Verification items for the finished model (mm, model axes). A direction names the side the tool comes from. Coordinates: 2 decimals unless noted, no trailing zeros. Order: outer loops, then holes, each group sorted by start corner. A loop starts at its lowest first (then second) coordinate and runs counter-clockwise, first axis right, second up. Notation, with made-up numbers: M 57.25,54.5 L 94.25,54.5 A35 cw 94.25,89.5 Z; hole C -3.75,25.5 d7. An arc over 180 degrees is marked long. Answer as a JSON object with one key per item and string values. Group by question number.
(1) Cross-section at A-A (y = 0). Enter the section's corners in (x, z), plus the area to 4 significant figures.
(2) Access from +Z, -Z, +X, -X, +Y, -Y to the whole of each face (thin tool, end or side, straight path). Record for faces 4 (the face through (-6.35, 0, -2)), 5 (the face through (0, -5, 2)), 6 (the face through (2, -6, 0)).
(3) Mould release check, pull along Z, two halves, no side actions. Record for faces 1 (the face through (0, -2, 13)), 2 (the face through (-2, 0, -5)), 3 (the face through (-0.54, -2.44, 8.44)): released by +Z, released by -Z, zero draft, split by the parting line, or undercut.
(4) Gauge pin test, flat ends, axial feed: pin 1 Ø4.5 at (x, y) = (0, 3) entering from +Z; pin 2 Ø8 at (x, z) = (-2, 8) entering from -Y; pin 3 Ø6 at (y, z) = (-3.5, 9) entering from -X; pin 4 Ø1.5 at (y, z) = (1, 6) entering from +X. Record the tip position at first contact, or that the pin passes through.
(5) Cross-section at B-B (x = 0). Enter the section's corners in (y, z), plus the area to 3 significant figures.
(6) Material ranges on line 1 (Y direction, x = 0, z = 11.1); line 2 (Z direction, x = -0.5, y = 4.75); line 3 (Z direction, x = 1.75, y = 6.25), recorded low to high.
(7) Cross-section at C-C (z = 0.75). Enter the section's corners in (x, y), plus the area to 3 significant figures.
from build123d import *

# Parameters (mm, degrees)
EXTRUDE_1_DEPTH     = 5
SKETCH_2_R          = 7.1
EXTRUDE_2_DEPTH     = 2
SKETCH_3_R          = 2.5
EXTRUDE_3_DEPTH     = 7
CHAMFER_1_SIZE      = 2
SKETCH_4_R          = 1.6
CUT_EXTRUDE_1_DEPTH = 30
CHAMFER_2_SIZE      = 1
MOVE_FACE_1_BY      = 4


with BuildPart() as part:
    # ｽｹｯﾁ1 → ﾎﾞｽ - 押し出し1 (new body)
    with BuildSketch(Plane.XY):
        with BuildLine():
            Line((-6.35, -0.875), (-6.036917674, -0.875))
            ThreePointArc((-6.036917674, -0.875), (6.1, 0), (-6.036917674, 0.875))
            Line((-6.036917674, 0.875), (-6.35, 0.875))
            Line((-6.35, 0.875), (-6.35, -0.875))
        make_face()
    extrude(amount=-EXTRUDE_1_DEPTH)

    # ｽｹｯﾁ2 → ﾎﾞｽ - 押し出し2 (add)
    with BuildSketch(Plane.XY):
        Circle(SKETCH_2_R)
    extrude(amount=EXTRUDE_2_DEPTH)

    # ｽｹｯﾁ3 → ﾎﾞｽ - 押し出し3 (add)
    with BuildSketch(Plane.XY.offset(2)):
        Circle(SKETCH_3_R)
    extrude(amount=EXTRUDE_3_DEPTH)

    # 面取り1
    chamfer_1_edges = [part.edges().sort_by_distance(p)[0] for p in [
        (-2.5, 0, 2),
    ]]
    chamfer(chamfer_1_edges, length=CHAMFER_1_SIZE)

    # ｽｹｯﾁ4 → ｶｯﾄ - 押し出し1 (cut)
    with BuildSketch(Plane.XY.offset(9)):
        Circle(SKETCH_4_R)
    extrude(amount=-CUT_EXTRUDE_1_DEPTH, mode=Mode.SUBTRACT)

    # 面取り2
    chamfer_2_edges = [part.edges().sort_by_distance(p)[0] for p in [
        (6.1, 0, -5),
    ]]
    chamfer(chamfer_2_edges, length=CHAMFER_2_SIZE)

    # Move Face 1: a face moved outward by 4.0
    extrude(part.faces().sort_by_distance((0, -2, 9))[0], amount=MOVE_FACE_1_BY, dir=(0, 0, 1))


solid = part.part
Taken from the geometry:
{
 "1": {"outline": "M -7.1,0 L -6.35,0 L -6.35,-5 L -1.6,-5 L -1.6,13 L -2.5,13 L -2.5,4 L -4.5,2 L -7.1,2 Z; M 1.6,-5 L 5.1,-5 L 6.1,-4 L 6.1,0 L 7.1,0 L 7.1,2 L 4.5,2 L 2.5,4 L 2.5,13 L 1.6,13 Z", "area": "91.55 mm²"},
 "2": {"face 4": "-Z, -X, +Y, -Y", "face 5": "+Z", "face 6": "-Z"},
 "3": {"face 1": "released by +Z", "face 2": "released by -Z", "face 3": "zero draft"},
 "4": {"pin 1": "stops at z = 13", "pin 2": "stops at y = -2.5", "pin 3": "stops at x = -2.45", "pin 4": "stops at x = 2.49"},
 "5": {"outline": "M -7.1,0 L -6.1,0 L -6.1,-4 L -5.1,-5 L -1.6,-5 L -1.6,13 L -2.5,13 L -2.5,4 L -4.5,2 L -7.1,2 Z; M 1.6,-5 L 5.1,-5 L 6.1,-4 L 6.1,0 L 7.1,0 L 7.1,2 L 4.5,2 L 2.5,4 L 2.5,13 L 1.6,13 Z", "area": "89.8 mm²"},
 "6": {"line 1": "y = -2.5 to -1.6, 1.6 to 2.5", "line 2": "z = -5 to 2", "line 3": "z = 0 to 2"},
 "7": {"outline": "C 0,0 d14.2; hole C 0,0 d3.2", "area": "150 mm²"}
}
